Here's the drawing with two shaded views (mm, measured from the low corner). I have some questions. A direction names the side the tool comes from. Round coordinates to 2 decimals unless told otherwise and drop trailing zeros. Write each loop counter-clockwise with the first axis right and the second up, starting at its lowest first coordinate (ties: lowest second). Pieces come first, ordered by that corner, then holes. Notation, with made-up numbers: (26, -24.75) -> (41, -24.75) arc R26 cw to (41, 13.25) -> close; hole circle Ø2 at (68, 70.25). An arc over 180 degrees is marked (long way). Use CSV: the item, a comma, the result in double quotes.
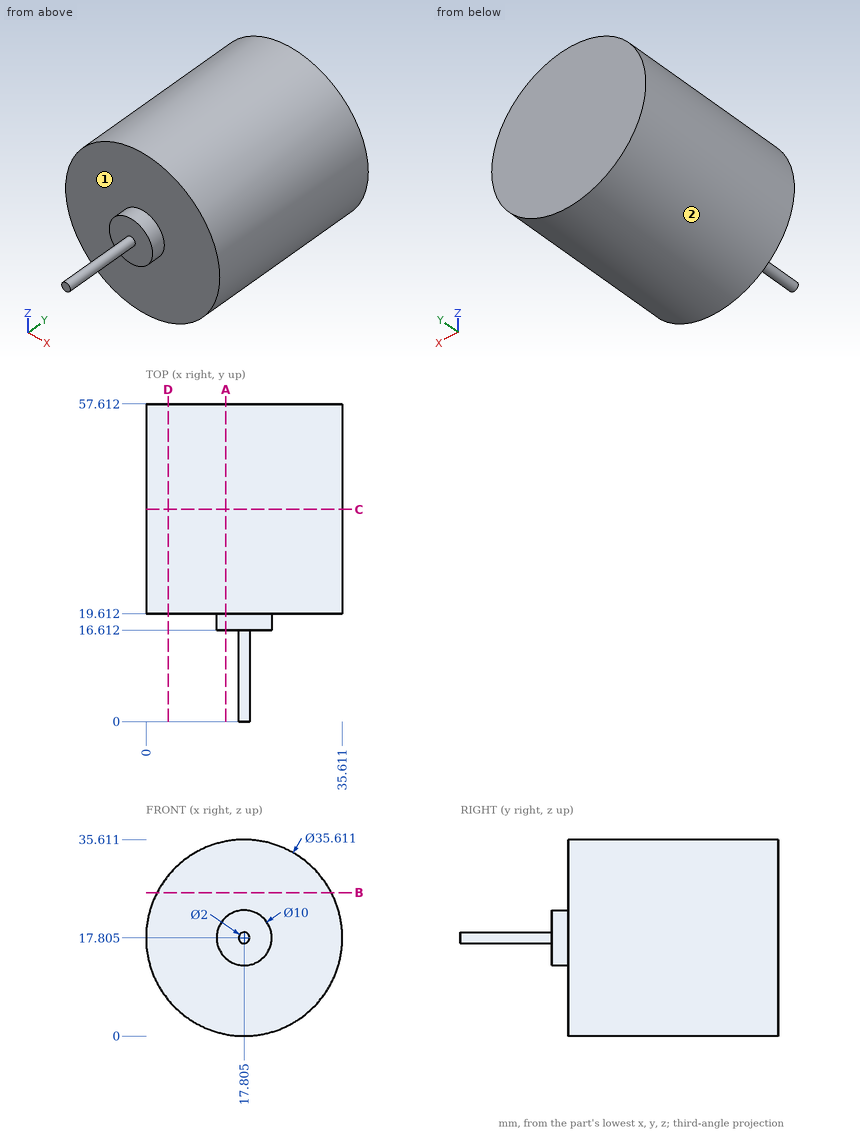
Q1. Suppose I cut it at D-D (x = 4). Write out the boundary of the cut face in (y, z).
Resolved:
outline,"(19.61, 6.56) -> (57.61, 6.56) -> (57.61, 29.05) -> (19.61, 29.05) -> close"
Q2. Please list where these lines run through material, in increasing order: probe 1 along X at (y, z) = (31, 18.5); probe 2 along Y at (x, z) = (13.5, 29); probe 3 along Y at (x, z) = (14, 15).
Resolved:
probe 1,"x = 0.01 to 35.6"
probe 2,"y = 19.61 to 57.61"
probe 3,"y = 16.61 to 57.61"
Q3. Suppose I cut it at A-A (x = 14.5). Write out the boundary of the cut face in (y, z).
Resolved:
outline,"(16.61, 14.05) -> (19.61, 14.05) -> (19.61, 0.31) -> (57.61, 0.31) -> (57.61, 35.3) -> (19.61, 35.3) -> (19.61, 21.56) -> (16.61, 21.56) -> close"
Q4. On a 3-axis mill with a long thin cutter (end or side, diameter ignored), from which of +Z, -Z, +X, -X, +Y, -Y can I reach the whole of each face in a straight line? I mean the marked faces 1 and 2. Say none if no direction works.
Resolved:
face 1,"-Y"
face 2,"+Y, -Y"
Q5. Suppose I cut it at B-B (z = 26). Write out the boundary of the cut face in (x, y).
Resolved:
outline,"(2, 19.61) -> (33.61, 19.61) -> (33.61, 57.61) -> (2, 57.61) -> close"
Q6. Will these pins go through, and if not, where does the flat tip stop? P1, Ø12, axis at y = 39, z = 15, coming from the -X side; P2, Ø8, axis at x = 25.5, y = 48, coming from the -Z side; P3, Ø6, axis at x = 28.5, z = 6.5, coming from the -Y side; P4, Ø8, axis at x = 13, y = 30.5, coming from the +Z side.
Resolved:
P1,"stops at x = 0"
P2,"stops at z = 0.39"
P3,"stops at y = 19.61"
P4,"stops at z = 35.59"
Q7. Suppose I cut it at C-C (y = 38.5). Write out the boundary of the cut face in (x, z) (1 decimal).
Resolved:
outline,"circle Ø35.6 at (17.8, 17.8)"
